Autodesk Inventor part; units mm, degrees
ref_plane "YZ Plane" through (0, 0, 0) normal (1, 0, 0) x (0, 1, 0)
ref_plane "XZ Plane" through (0, 0, 0) normal (0, 1, 0) x (-1, 0, 0)
ref_plane "XY Plane" through (0, 0, 0) normal (0, 0, 1) x (1, 0, 0)
sketch "スケッチ1" plane through (0, 0, 0) normal (0, 0, 1) x (1, 0, 0)
  line L0 (0, 0) -> (100, 0)
  line L1 (100, 0) -> (100, 120)
  line L2 (100, 120) -> (0, 120)
  line L3 (0, 120) -> (0, 0)
  line L4 (0, 10) -> (100, 10) construction
  circle A0 centre (10, 10) radius 2.5
  circle A1 centre (90, 10) radius 2.5
  circle A2 centre (10, 110) radius 4
  circle A3 centre (10, 30) radius 4
  circle A4 centre (90, 110) radius 4
  circle A5 centre (90, 30) radius 4
  line L5 (10, 110) -> (10, 30) construction
  line L6 (10, 30) -> (90, 30) construction
  line L7 (90, 30) -> (90, 110) construction
  line L8 (90, 110) -> (10, 110) construction
  dimension "d0" = 5
  dimension "d1" = 10
  dimension "d2" = 10
  dimension "d3" = 10
  dimension "d4" = 100
  dimension "d5" = 120
  dimension "d12" = 8
  dimension "d13" = 10
  dimension "d14" = 10
  dimension "d15" = 10
  dimension "d16" = 10
  dimension "d21" = 80
extrude "押し出し1" add sketch "スケッチ1" along normal blind 3
fillet "フィレット1" radius 5 4 edges at (100, 120, 1.5) (0, 120, 1.5) (100, 0, 1.5) (0, 0, 1.5)
properties part number "LRFマウント"
Verification items for the finished model (mm, model axes). Coordinates: 2 decimals unless noted, no trailing zeros. Write each loop counter-clockwise with the first axis right and the second up, starting at its lowest first coordinate (ties: lowest second). Pieces come first, ordered by that corner, then holes. Notation, with made-up numbers: M 11.5,-34.75 L 23.5,-34.75 A8 ccw 23.5,-27.75 Z; hole C 18.5,-11 d5. An arc over 180 degrees is marked long. Use a Markdown table: item, result.
Q1. Sectioned sample at D-D, the plane y = 10. Record the boundary of the cut face in (x, z), plus the area to 3 significant figures.
Reply:
| item | result |
|---|---|
| outline | M 0,0 L 7.5,0 L 7.5,3 L 0,3 Z; M 12.5,0 L 87.5,0 L 87.5,3 L 12.5,3 Z; M 92.5,0 L 100,0 L 100,3 L 92.5,3 Z |
| area | 270 mm² |
Q2. Go/stop test with a flat-tipped pin: P1, Ø13, axis at x = 90, y = 30, coming from the -Z side. Record where the tip stops, or that it passes through.
Reply:
| item | result |
|---|---|
| P1 | stops at z = 0 |
Q3. Draft check along Y on faces 1 (the face through (99, 118, 2)), 2 (the face through (1, 2, 2)), 3 (the face through (49, 61, 3)), 4 (the face through (88, 11.5, 1.5)). Enter one of: +Y half, -Y half, draft (parallel to the pull), parting line (faces both ways), or undercut.
Reply:
| item | result |
|---|---|
| face 1 | +Y half |
| face 2 | -Y half |
| face 3 | draft |
| face 4 | undercut |
Q4. Thickness scan on line 1 (Y direction, x = 90, z = 2.25); line 2 (X direction, y = 109.5, z = 1.45); line 3 (Y direction, x = 6.5, z = 2.85). Record the ranges inside material, lowest first.
Reply:
| item | result |
|---|---|
| line 1 | y = 0 to 7.5, 12.5 to 26, 34 to 106, 114 to 120 |
| line 2 | x = 0 to 6.03, 13.97 to 86.03, 93.97 to 100 |
| line 3 | y = 0 to 28.06, 31.94 to 108.06, 111.94 to 120 |
Q5. Sectioned sample at C-C, the plane z = 0.7. Record the boundary of the cut face in (x, y), plus the area to 3 significant figures.
Reply:
| item | result |
|---|---|
| outline | M 0,5 A5 ccw 5,0 L 95,0 A5 ccw 100,5 L 100,115 A5 ccw 95,120 L 5,120 A5 ccw 0,115 Z; hole C 10,30 d8; hole C 10,110 d8; hole C 10,10 d5; hole C 90,30 d8; hole C 90,110 d8; hole C 90,10 d5 |
| area | 11,700 mm² |
Q6. Sectioned sample at B-B, the plane x = 90. Record the boundary of the cut face in (y, z).
Reply:
| item | result |
|---|---|
| outline | M 0,0 L 7.5,0 L 7.5,3 L 0,3 Z; M 12.5,0 L 26,0 L 26,3 L 12.5,3 Z; M 34,0 L 106,0 L 106,3 L 34,3 Z; M 114,0 L 120,0 L 120,3 L 114,3 Z |
Q7. Sectioned sample at A-A, the plane y = 30. Record the boundary of the cut face in (x, z), plus the area to 3 significant figures.
Reply:
| item | result |
|---|---|
| outline | M 0,0 L 6,0 L 6,3 L 0,3 Z; M 14,0 L 86,0 L 86,3 L 14,3 Z; M 94,0 L 100,0 L 100,3 L 94,3 Z |
| area | 252 mm² |
